Here's how the part is built. I have some questions about the finished solid (model axes, mm). A direction names the side the tool comes from. Coordinates: 2 decimals unless noted, no trailing zeros.
(1) Please list where these lines run through material, in increasing order: probe 1 along X at (y, z) = (0.75, -35.5); probe 2 along Z at (x, y) = (74.5, 3.5); probe 3 along X at (y, z) = (0.5, -8).
(2) Thinking about a two-plate mould opening in Z: for faces 3 (the cylindrical face through (48.133, 3.422, -8.759)), 4 (the flat face through (-1, 5, -1)), 5 (the cylindrical face through (77.797, 2.535, -66.859)), which applies, released by +Z, released by -Z, zero draft, split by the parting line, or undercut?
(3) For pin 1 Ø1.8 at (x, z) = (-72.5, -63.5) entering from -Y; pin 2 Ø5.5 at (x, z) = (24, 35.55) entering from +Y, each with a flat end and sliding along its axis, tell me the tip position at first contact or that it passes through.
(4) Which directions (+Z, -Z, +X, -X, +Y, -Y) give clear straight access to the entire face, cutting with the end or side of a thin tool? Please do faces 1 (the flat face through (6, 1.8, -36)), 2 (the cylindrical face through (-77.859, 2.535, -66.797)).
```python
from build123d import *

# Parameters (mm, degrees)
SKETCH8_W           = 158
SKETCH8_H           = 136
SKETCH8_R           = 1.5
BOSS_EXTRUDE4_DEPTH = 5
FILLET2_R           = 4
SKETCH10_R          = 1.5
CUT_EXTRUDE5_DEPTH  = 5
SKETCH11_R          = 3.5
CUT_EXTRUDE6_DEPTH  = 3.2


with BuildPart() as part:
    # Sketch8 → Boss-Extrude4 (new body)
    with BuildSketch(Plane(origin=(0, 0, 0), x_dir=(1, 0, 0), z_dir=(0, 1, 0))):
        Rectangle(SKETCH8_W, SKETCH8_H)
        with Locations(Location((74.5, 63.5, 0), (0, 0, 270))):
            Circle(SKETCH8_R, mode=Mode.SUBTRACT)
        with Locations(Location((-72.5, 63.5, 0), (0, 0, 270))):
            Circle(SKETCH8_R, mode=Mode.SUBTRACT)
        with Locations(Location((-72.5, -63.5, 0), (0, 0, 90))):
            Circle(SKETCH8_R, mode=Mode.SUBTRACT)
        with Locations(Location((74.5, -63.5, 0), (0, 0, 90))):
            Circle(SKETCH8_R, mode=Mode.SUBTRACT)
    extrude(amount=BOSS_EXTRUDE4_DEPTH)

    # Fillet2
    fillet2_edges = [part.edges().sort_by_distance(p)[0] for p in [
        (79, 2.5, 68),
        (-79, 2.5, 68),
        (-79, 2.5, -68),
        (79, 2.5, -68),
    ]]
    fillet(fillet2_edges, radius=FILLET2_R)

    # Sketch10 → Cut-Extrude5 (cut)
    with BuildSketch(Plane(origin=(0, 5, 0), x_dir=(1, 0, 0), z_dir=(0, 1, 0))):
        with Locations(Location((24, 35.55, 0), (0, 0, 270))):
            Circle(SKETCH10_R)
        with Locations(Location((24, -35.55, 0), (0, 0, 90))):
            Circle(SKETCH10_R)
        with Locations(Location((8, -35.55, 0), (0, 0, 270))):
            Circle(SKETCH10_R)
        with Locations(Location((8, 35.55, 0), (0, 0, 90))):
            Circle(SKETCH10_R)
        with Locations(Location((51.55, -8, 0), (0, 0, 270))):
            Circle(SKETCH10_R)
        with Locations(Location((51.55, 8, 0), (0, 0, 90))):
            Circle(SKETCH10_R)
    extrude(amount=-CUT_EXTRUDE5_DEPTH, mode=Mode.SUBTRACT)

    # Sketch11 → Cut-Extrude6 (cut)
    with BuildSketch(Plane(origin=(0, 5, 0), x_dir=(1, 0, 0), z_dir=(0, 1, 0))):
        with Locations(Location((24, 35.55, 0), (0, 0, 270))):
            Circle(SKETCH11_R)
        with Locations(Location((8, 35.55, 0), (0, 0, 270))):
            Circle(SKETCH11_R)
        with Locations(Location((51.55, 8, 0), (0, 0, 270))):
            Circle(SKETCH11_R)
        with Locations(Location((51.55, -8, 0), (0, 0, 270))):
            Circle(SKETCH11_R)
        with Locations(Location((24, -35.55, 0), (0, 0, 270))):
            Circle(SKETCH11_R)
        with Locations(Location((8, -35.55, 0), (0, 0, 270))):
            Circle(SKETCH11_R)
    extrude(amount=-CUT_EXTRUDE6_DEPTH, mode=Mode.SUBTRACT)


solid = part.part
```
Recorded:
1. probe 1: x = -79 to 6.5, 9.5 to 22.5, 25.5 to 79
1. probe 2: z = -68 to -65, -62 to 62, 65 to 68
1. probe 3: x = -79 to 50.05, 53.05 to 79
2. face 3: undercut
2. face 4: zero draft
2. face 5: released by -Z
3. pin 1: passes through
3. pin 2: stops at y = 1.8
4. face 1: +Y
4. face 2: -Z, -X, +Y, -Y
